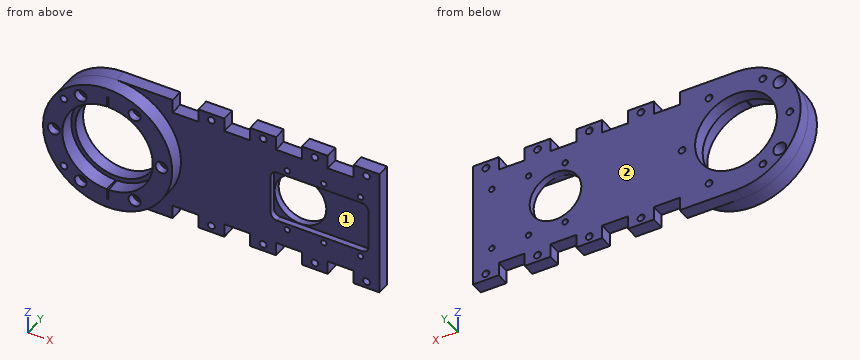
from build123d import *

# Parameters (mm, degrees)
SKETCH1_W           = 55.6
SKETCH1_H           = 35.6
SKETCH1_R           = 1.3
SKETCH1_W_2         = 45.4
SKETCH1_H_2         = 24.4
BOSS_EXTRUDE1_DEPTH = 2.8
BOSS_EXTRUDE2_START = 3.2
SKETCH1_5_W         = 55.6
SKETCH1_5_H         = 35.6
SKETCH1_5_R         = 1.3
SKETCH1_5_W_2       = 45.4
SKETCH1_5_H_2       = 24.4
SKETCH1_5_R_2       = 12
BOSS_EXTRUDE2_DEPTH = 3.2
FILLET1_R           = 3
BOSS_EXTRUDE3_START = -2.8
SKETCH2_R           = 19
BOSS_EXTRUDE3_DEPTH = 6
BOSS_EXTRUDE4_START = -7
SKETCH3_R           = 30
BOSS_EXTRUDE4_DEPTH = 7
SKETCH4_R           = 1.6
CUT_EXTRUDE1_DEPTH  = 119.413327375
SKETCH5_R           = 2.8
CUT_EXTRUDE2_DEPTH  = 3.5
BOSS_EXTRUDE5_START = -6
BOSS_EXTRUDE5_DEPTH = 6
SKETCH7_W           = 12
SKETCH7_H           = 6.35
CUT_EXTRUDE3_DEPTH  = 118.905538886
SKETCH8_R           = 1.6
CUT_EXTRUDE4_DEPTH  = 118.905538886
SKETCH9_R           = 1.6
CUT_EXTRUDE5_DEPTH  = 119.413327375
SKETCH10_R          = 3
CUT_EXTRUDE7_DEPTH  = 7


with BuildPart() as part:
    # Sketch1 → Boss-Extrude1 (new body)
    with BuildSketch(Plane(origin=(0, 0, 0), x_dir=(1, 0, 0), z_dir=(0, 1, 0))):
        with Locations((10.5, 0)):
            Rectangle(SKETCH1_W, SKETCH1_H)
        with Locations(Location((12.5, -15, 0), (0, 0, 270))):
            Circle(SKETCH1_R, mode=Mode.SUBTRACT)
        with Locations(Location((-4.5, 15, 0), (0, 0, 270))):
            Circle(SKETCH1_R, mode=Mode.SUBTRACT)
        with Locations(Location((12.5, 15, 0), (0, 0, 270))):
            Circle(SKETCH1_R, mode=Mode.SUBTRACT)
        with Locations(Location((29.5, 15, 0), (0, 0, 270))):
            Circle(SKETCH1_R, mode=Mode.SUBTRACT)
        with Locations(Location((29.5, -15, 0), (0, 0, 270))):
            Circle(SKETCH1_R, mode=Mode.SUBTRACT)
        with Locations(Location((-4.5, -15, 0), (0, 0, 270))):
            Circle(SKETCH1_R, mode=Mode.SUBTRACT)
        with Locations((10.5, 0)):
            Rectangle(SKETCH1_W_2, SKETCH1_H_2, mode=Mode.SUBTRACT)
    extrude(amount=-BOSS_EXTRUDE1_DEPTH)

    # Sketch1<5> → Boss-Extrude2 (add)
    # profile 1 of 2: a face of its own
    with BuildSketch(Plane(origin=(0, 0, 0), x_dir=(1, 0, 0), z_dir=(0, 1, 0)).offset(BOSS_EXTRUDE2_START)):
        with Locations((10.5, 0)):
            Rectangle(SKETCH1_5_W, SKETCH1_5_H)
        with Locations(Location((12.5, -15, 0), (0, 0, 270))):
            Circle(SKETCH1_5_R, mode=Mode.SUBTRACT)
        with Locations(Location((-4.5, 15, 0), (0, 0, 270))):
            Circle(SKETCH1_5_R, mode=Mode.SUBTRACT)
        with Locations(Location((12.5, 15, 0), (0, 0, 270))):
            Circle(SKETCH1_5_R, mode=Mode.SUBTRACT)
        with Locations(Location((29.5, 15, 0), (0, 0, 270))):
            Circle(SKETCH1_5_R, mode=Mode.SUBTRACT)
        with Locations(Location((29.5, -15, 0), (0, 0, 270))):
            Circle(SKETCH1_5_R, mode=Mode.SUBTRACT)
        with Locations(Location((-4.5, -15, 0), (0, 0, 270))):
            Circle(SKETCH1_5_R, mode=Mode.SUBTRACT)
        with Locations((10.5, 0)):
            Rectangle(SKETCH1_5_W_2, SKETCH1_5_H_2, mode=Mode.SUBTRACT)
    # profile 2 of 2: a face of its own
    with BuildSketch(Plane(origin=(0, 0, 0), x_dir=(1, 0, 0), z_dir=(0, 1, 0)).offset(BOSS_EXTRUDE2_START)):
        with Locations((10.5, 0)):
            Rectangle(SKETCH1_5_W_2, SKETCH1_5_H_2)
        with Locations(Location((0, 0, 0), (0, 0, 270))):
            Circle(SKETCH1_5_R_2, mode=Mode.SUBTRACT)
    extrude(amount=-BOSS_EXTRUDE2_DEPTH)

    # Fillet1
    fillet1_edges = [part.edges().sort_by_distance(p)[0] for p in [
        (-12.2, -1.4, -12.2),
        (-12.2, -1.4, 12.2),
        (33.2, -1.4, 12.2),
        (33.2, -1.4, -12.2),
    ]]
    fillet(fillet1_edges, radius=FILLET1_R)

    # Sketch2 → Boss-Extrude3 (add)
    with BuildSketch(Plane(origin=(0, 0, 0), x_dir=(1, 0, 0), z_dir=(0, 1, 0)).offset(BOSS_EXTRUDE3_START)):
        with BuildLine():
            Line((-17.3, 17.8), (-59.661294031, 17.8))
            ThreePointArc((-59.661294031, 17.8), (-113.81, 0), (-59.661294031, -17.8))
            Line((-59.661294031, -17.8), (-17.3, -17.8))
            Line((-17.3, -17.8), (-17.3, 17.8))
        make_face()
        with Locations(Location((-83.81, 0, 0), (0, 0, 270))):
            Circle(SKETCH2_R, mode=Mode.SUBTRACT)
    extrude(amount=BOSS_EXTRUDE3_DEPTH)

    # Sketch3 → Boss-Extrude4 (add)
    with BuildSketch(Plane(origin=(0, -2.8, 0), x_dir=(1, 0, 0), z_dir=(0, 1, 0)).offset(BOSS_EXTRUDE4_START)):
        with Locations(Location((-83.81, 0, 0), (0, 0, 36.393910191))):
            Circle(SKETCH3_R)
        with BuildLine():
            Line((-84.185, 20.996651519), (-84.185, 25.996651519))
            Line((-84.185, 25.996651519), (-83.435, 25.996651519))
            Line((-83.435, 25.996651519), (-83.435, 20.996651519))
            ThreePointArc((-83.435, 20.996651519), (-62.81, 0), (-83.435, -20.996651519))
            Line((-83.435, -20.996651519), (-83.435, -25.996651519))
            Line((-83.435, -25.996651519), (-84.185, -25.996651519))
            Line((-84.185, -25.996651519), (-84.185, -20.996651519))
            ThreePointArc((-84.185, -20.996651519), (-104.81, 0), (-84.185, 20.996651519))
        make_face(mode=Mode.SUBTRACT)
    extrude(amount=BOSS_EXTRUDE4_DEPTH)

    # Sketch4 → Cut-Extrude1 (cut, through all)
    with BuildSketch(Plane(origin=(0, 3.2, 0), x_dir=(1, 0, 0), z_dir=(0, 1, 0))):
        with Locations(Location((-58.81, 0, 0), (0, 0, 270))):
            Circle(SKETCH4_R)
        with Locations(Location((-71.31, -21.650635095, 0), (0, 0, 270))):
            Circle(SKETCH4_R)
        with Locations(Location((-96.31, -21.650635095, 0), (0, 0, 270))):
            Circle(SKETCH4_R)
        with Locations(Location((-108.81, 0, 0), (0, 0, 270))):
            Circle(SKETCH4_R)
        with Locations(Location((-96.31, 21.650635095, 0), (0, 0, 270))):
            Circle(SKETCH4_R)
        with Locations(Location((-71.31, 21.650635095, 0), (0, 0, 270))):
            Circle(SKETCH4_R)
    extrude(amount=-CUT_EXTRUDE1_DEPTH, mode=Mode.SUBTRACT)

    # Sketch5 → Cut-Extrude2 (cut)
    with BuildSketch(Plane(origin=(0, -9.8, 0), x_dir=(-1, 0, 0), z_dir=(0, -1, 0))):
        with Locations(Location((96.31, 21.650635095, 0), (0, 0, 90))):
            Circle(SKETCH5_R)
        with Locations(Location((108.81, 0, 0), (0, 0, 90))):
            Circle(SKETCH5_R)
        with Locations(Location((96.31, -21.650635095, 0), (0, 0, 90))):
            Circle(SKETCH5_R)
        with Locations(Location((71.31, -21.650635095, 0), (0, 0, 90))):
            Circle(SKETCH5_R)
        with Locations(Location((58.81, 0, 0), (0, 0, 90))):
            Circle(SKETCH5_R)
        with Locations(Location((71.31, 21.650635095, 0), (0, 0, 90))):
            Circle(SKETCH5_R)
    extrude(amount=-CUT_EXTRUDE2_DEPTH, mode=Mode.SUBTRACT)

    # Sketch6 → Boss-Extrude5 (add)
    with BuildSketch(Plane(origin=(0, 3.2, 0), x_dir=(1, 0, 0), z_dir=(0, 1, 0)).offset(BOSS_EXTRUDE5_START)):
        with BuildLine():
            Line((38.3, 17.8), (38.3, 30))
            Line((38.3, 30), (-83.81, 30))
            ThreePointArc((-83.81, 30), (-70.282250742, 26.776855678), (-59.661294031, 17.8))
            Line((-59.661294031, 17.8), (38.3, 17.8))
        make_face()
    boss_extrude5 = extrude(amount=BOSS_EXTRUDE5_DEPTH)

    # Mirror1: Boss-Extrude5 across plane
    add(boss_extrude5.mirror(Plane.XY))

    # Sketch7 → Cut-Extrude3 (cut, through all)
    with BuildSketch(Plane.XZ.offset(2.8)):
        with Locations((20.3, -26.825)):
            Rectangle(SKETCH7_W, SKETCH7_H)
        with Locations((-3.7, -26.825)):
            Rectangle(SKETCH7_W, SKETCH7_H)
        with Locations((-27.7, -26.825)):
            Rectangle(SKETCH7_W, SKETCH7_H)
        with Locations((-51.7, -26.825)):
            Rectangle(SKETCH7_W, SKETCH7_H)
    cut_extrude3 = extrude(amount=-CUT_EXTRUDE3_DEPTH, mode=Mode.SUBTRACT)

    # Mirror2: Cut-Extrude3 across plane
    add(cut_extrude3.mirror(Plane.XY), mode=Mode.SUBTRACT)

    # Sketch8 → Cut-Extrude4 (cut, through all)
    with BuildSketch(Plane.XZ.offset(2.8)):
        with Locations(Location((-39.7, -26.825, 0), (0, 0, 270))):
            Circle(SKETCH8_R)
        with Locations(Location((-15.7, -26.825, 0), (0, 0, 270))):
            Circle(SKETCH8_R)
        with Locations(Location((8.3, -26.825, 0), (0, 0, 270))):
            Circle(SKETCH8_R)
        with Locations(Location((32.3, -26.825, 0), (0, 0, 270))):
            Circle(SKETCH8_R)
    cut_extrude4 = extrude(amount=-CUT_EXTRUDE4_DEPTH, mode=Mode.SUBTRACT)

    # Mirror3: Cut-Extrude4 across plane
    add(cut_extrude4.mirror(Plane.XY), mode=Mode.SUBTRACT)

    # Sketch9 → Cut-Extrude5 (cut, through all)
    with BuildSketch(Plane(origin=(0, 3.2, 0), x_dir=(1, 0, 0), z_dir=(0, 1, 0))):
        with Locations(Location((-104.110177743, -17.033871657, 0), (0, 0, 270))):
            Circle(SKETCH9_R)
        with Locations(Location((-104.110177743, 17.033871657, 0), (0, 0, 270))):
            Circle(SKETCH9_R)
    extrude(amount=-CUT_EXTRUDE5_DEPTH, mode=Mode.SUBTRACT)

    # Sketch10 → Cut-Extrude7 (cut)
    with BuildSketch(Plane(origin=(0, 3.2, 0), x_dir=(1, 0, 0), z_dir=(0, 1, 0))):
        with Locations(Location((-104.110177743, 17.033871657, 0), (0, 0, 270))):
            Circle(SKETCH10_R)
        with Locations(Location((-104.110177743, -17.033871657, 0), (0, 0, 270))):
            Circle(SKETCH10_R)
    extrude(amount=-CUT_EXTRUDE7_DEPTH, mode=Mode.SUBTRACT)


solid = part.part
Geometry: final body of the model. Coordinates: model frame, mm. Face numbers are marked on the shaded views. Coordinates: 2 decimals unless noted, no trailing zeros. Order: outer loops, then holes, each group sorted by start corner. A loop starts at its lowest first (then second) coordinate and runs counter-clockwise, first axis right, second up.
(1) Section query A-A (x = 0). Return the cut outline in (y, z), plus the area to 3 significant figures.
(2) First-contact query: pin 1 (3 mm diameter, centred on x = -53.5, y = -1, fed in from -Z); pin 2 (2 mm diameter, centred on y = -6.5, z = -11.5, fed in from -X); pin 3 (3 mm diameter, centred on x = 12.5, z = -15, fed in from -Y). Flat tips, straight axial feed; report the tip coordinate or a pass-through.
(3) Material intervals for probe 1 along X at (y, z) = (0.75, 0); probe 2 along X at (y, z) = (-1.45, 15); probe 3 along Z at (x, y) = (-96.31, -3.75), sorted ascending.
(4) Draft query along X for the marked faces 1 and 2. Return one class per face: pulls with the +X half, pulls with the -X half, needs draft (parallel to the pull), parting line crosses it, or undercut.
(5) Section query C-C (x = -71.31). State how many separate pieces and enclosed holes the cut face has, plus the area to 3 significant figures.
(6) Section query B-B (z = -6.5). Return the cut outline in (x, y).
(7) Section query D-D (x = -108.81). Return the cut outline in (y, z), plus the area to 3 significant figures.
Solution:
1. outline: (-2.8, -23.65) - (3.2, -23.65) - (3.2, -12) - (0, -12) - (0, -12.2) - (-2.8, -12.2) - close; (-2.8, 12.2) - (0, 12.2) - (0, 12) - (3.2, 12) - (3.2, 23.65) - (-2.8, 23.65) - close
1. area: 139 mm2
2. pin 1: stops at z = -23.65
2. pin 2: stops at x = -111.91
2. pin 3: stops at y = -2.8
3. probe 1: x = -113.81 to -110.41, -107.21 to -102.81, -64.81 to -60.41, -57.21 to -12, 12 to 38.3
3. probe 2: x = -109.79 to -106.32, -101.9 to -95.47, -72.15 to -5.8, -3.2 to 11.2, 13.8 to 28.2, 30.8 to 38.3
3. probe 3: z = -27.27 to -23.25, -20.05 to -16.87, 16.87 to 20.05, 23.25 to 27.27
4. face 1: undercut
4. face 2: needs draft
5. separate pieces: 4
5. enclosed holes: 0
5. area: 234 mm2
6. outline: (-113.1, -9.8) - (-103.78, -9.8) - (-103.78, -2.8) - (-101.66, -2.8) - (-101.66, 3.2) - (-113.1, 3.2) - close; (-65.96, -2.8) - (-63.84, -2.8) - (-63.84, -9.8) - (-54.52, -9.8) - (-54.52, -2.8) - (-12.2, -2.8) - (-12.2, 0) - (-10.09, 0) - (-10.09, 3.2) - (-65.96, 3.2) - close; (10.09, 0) - (33.2, 0) - (33.2, -2.8) - (38.3, -2.8) - (38.3, 3.2) - (10.09, 3.2) - close
7. outline: (-9.8, -16.58) - (3.2, -16.58) - (3.2, -1.6) - (-6.3, -1.6) - (-6.3, -2.8) - (-9.8, -2.8) - close; (-9.8, 2.8) - (-6.3, 2.8) - (-6.3, 1.6) - (3.2, 1.6) - (3.2, 16.58) - (-9.8, 16.58) - close
7. area: 381 mm2
